from build123d import *

# Parameters (mm, degrees)
SKETCH_W        = 76.2
SKETCH_H        = 76.2
PAD_DEPTH       = 4
SKETCH001_R     = 25.4
POCKET_DEPTH    = 4.001
SKETCH002_R     = 2.25
POCKET001_DEPTH = 4.001
SKETCH003_R     = 30.4
SKETCH003_R_2   = 25.4
PAD001_DEPTH    = 25
SKETCH004_R     = 30.4
PAD002_DEPTH    = 3
SKETCH005_W     = 6
SKETCH005_H     = 11
POCKET002_DEPTH = 32.001
SKETCH006_W     = 5
SKETCH006_H     = 38
PAD003_DEPTH    = 42
POCKET003_DEPTH = 33.351
FILLET_R        = 1.5
FILLET001_R     = 3
FILLET002_R     = 0.4
FILLET003_R     = 3
FILLET004_R     = 6


with BuildPart() as part:
    # Sketch → Pad (new body)
    with BuildSketch(Plane.XY):
        Rectangle(SKETCH_W, SKETCH_H)
    extrude(amount=PAD_DEPTH)

    # Sketch001 (on Face6 of Pad) → Pocket (cut, through all)
    with BuildSketch(Plane.XY.offset(4)):
        Circle(SKETCH001_R)
    extrude(amount=-POCKET_DEPTH, mode=Mode.SUBTRACT)

    # Sketch002 (on Face5 of Pocket) → Pocket001 (cut, through all)
    with BuildSketch(Plane.XY.offset(4)):
        with Locations((-30.1, -30.1)):
            Circle(SKETCH002_R)
        with Locations((30.1, -30.1)):
            Circle(SKETCH002_R)
        with Locations((30.1, 30.1)):
            Circle(SKETCH002_R)
        with Locations((-30.1, 30.1)):
            Circle(SKETCH002_R)
    extrude(amount=-POCKET001_DEPTH, mode=Mode.SUBTRACT)

    # Sketch003 (on Face5 of Pocket001) → Pad001 (join)
    with BuildSketch(Plane.XY.offset(4)):
        Circle(SKETCH003_R)
        Circle(SKETCH003_R_2, mode=Mode.SUBTRACT)
    extrude(amount=PAD001_DEPTH)

    # Sketch004 (on Face14 of Pad001) → Pad002 (join)
    with BuildSketch(Plane.XY.offset(29)):
        Circle(SKETCH004_R)
    extrude(amount=PAD002_DEPTH)

    # Sketch005 (on Face16 of Pad002) → Pocket002 (cut, through all)
    with BuildSketch(Plane.XY.offset(32)):
        Rectangle(SKETCH005_W, SKETCH005_H)
    extrude(amount=-POCKET002_DEPTH, mode=Mode.SUBTRACT)

    # Sketch006 (on Face16 of Pocket002) → Pad003 (join)
    with BuildSketch(Plane.XY.offset(32)):
        with Locations((7.25, -8)):
            Rectangle(SKETCH006_W, SKETCH006_H)
    extrude(amount=PAD003_DEPTH)

    # CopySketch007 (on Face21 of Pad003) → Pocket003 (cut, through all)
    with BuildSketch(Plane(origin=(4.75, 0, 0), x_dir=(0, -1, 0), z_dir=(-1, 0, 0))):
        with BuildLine():
            ThreePointArc((-5.25, 45.013309), (-3, 42.763309), (-0.75, 45.013309))
            Line((-0.75, 45.013309), (-0.75, 70.013309))
            ThreePointArc((-0.75, 70.013309), (-3, 72.263309), (-5.25, 70.013309))
            Line((-5.25, 45.013309), (-5.25, 70.013309))
        make_face()
        with BuildLine():
            ThreePointArc((17.25, 35.513309), (19.5, 33.263309), (21.75, 35.513309))
            Line((21.75, 35.513309), (21.75, 60.513309))
            ThreePointArc((21.75, 60.513309), (19.5, 62.763309), (17.25, 60.513309))
            Line((17.25, 35.513309), (17.25, 60.513309))
        make_face()
    extrude(amount=-POCKET003_DEPTH, mode=Mode.SUBTRACT)

    # Fillet
    fillet_edges = [part.edges().sort_by_distance(p)[0] for p in [
        (4.75, -8, 32),
    ]]
    fillet(fillet_edges, radius=FILLET_R)

    # Fillet001
    fillet001_edges = [part.edges().sort_by_distance(p)[0] for p in [
        (9.75, -8, 32),
    ]]
    fillet(fillet001_edges, radius=FILLET001_R)

    # Fillet002
    fillet002_edges = [part.edges().sort_by_distance(p)[0] for p in [
        (7.25, -27, 32),
    ]]
    fillet(fillet002_edges, radius=FILLET002_R)

    # Fillet003
    fillet003_edges = [part.edges().sort_by_distance(p)[0] for p in [
        (7.25, 11, 32),
    ]]
    fillet(fillet003_edges, radius=FILLET003_R)

    # Fillet004
    fillet004_edges = [part.edges().sort_by_distance(p)[0] for p in [
        (7.25, -27, 74),
        (7.25, 11, 74),
    ]]
    fillet(fillet004_edges, radius=FILLET004_R)


solid = part.part
Verification items for the finished model (mm, model axes). A direction names the side the tool comes from. Coordinates: 2 decimals unless noted, no trailing zeros. Write each loop counter-clockwise with the first axis right and the second up, starting at its lowest first coordinate (ties: lowest second). Pieces come first, ordered by that corner, then holes. Notation, with made-up numbers: M -27,43 L 8,43 A15 ccw 8,53 Z; hole C 25,75.5 d3. An arc over 180 degrees is marked long. Use a Markdown table: item, result.
Q1. Thickness scan on line 1 (X direction, y = -30, z = 1); line 2 (Y direction, x = 8, z = 47). Record the ranges inside material, lowest first.
Reply:
| item | result |
|---|---|
| line 1 | x = -38.1 to -32.35, -27.85 to 27.85, 32.35 to 38.1 |
| line 2 | y = -27 to -21.75, -17.25 to 0.75, 5.25 to 11 |
Q2. Sectioned sample at C-C, the plane y = 3. Record the boundary of the cut face in (x, z), plus the area to 3 significant figures.
Reply:
| item | result |
|---|---|
| outline | M -38.1,0 L -25.22,0 L -25.22,29 L -3,29 L -3,32 L -30.25,32 L -30.25,4 L -38.1,4 Z; M 3,29 L 25.22,29 L 25.22,0 L 38.1,0 L 38.1,4 L 30.25,4 L 30.25,32 L 12.75,32 A3 cw 9.75,35 L 9.75,42.76 L 4.75,42.76 L 4.75,33.5 A1.5 cw 3.25,32 L 3,32 Z; M 4.75,72.26 L 9.75,72.26 L 9.75,74 L 4.75,74 Z |
| area | 583 mm² |
Q3. Draft check along X on faces 1 (the face through (7.285, 9.196, 72.289)), 2 (the face through (29.81, -27.87, 2.03)), 3 (the face through (-30.37, 1.34, 17.8)). Enter one of: +X half, -X half, draft (parallel to the pull), parting line (faces both ways), or undercut.
Reply:
| item | result |
|---|---|
| face 1 | draft |
| face 2 | undercut |
| face 3 | parting line |
Q4. Sectioned sample at A-A, the plane x = 0. Record the boundary of the cut face in (y, z).
Reply:
| item | result |
|---|---|
| outline | M -38.1,0 L -25.4,0 L -25.4,29 L -5.5,29 L -5.5,32 L -30.4,32 L -30.4,4 L -38.1,4 Z; M 5.5,29 L 25.4,29 L 25.4,0 L 38.1,0 L 38.1,4 L 30.4,4 L 30.4,32 L 5.5,32 Z |
Q5. Sectioned sample at B-B, the plane z = 41.5. Record the boundary of the cut face in (x, y), plus the area to 4 significant figures.
Reply:
| item | result |
|---|---|
| outline | M 4.75,-27 L 9.75,-27 L 9.75,-21.75 L 4.75,-21.75 Z; M 4.75,-17.25 L 9.75,-17.25 L 9.75,11 L 4.75,11 Z |
| area | 167.5 mm² |
Q6. Go/stop test with flat-tipped pins: P1, Ø5, axis at x = 5, z = 59, coming from the -Y side; P2, Ø0.9, axis at y = 0, z = 31, coming from the +X side; P3, Ø1, axis at x = -21.5, z = 8.5, coming from the +Y side; P4, Ø3, axis at x = -25.5, y = -21, coming from the -Z side. Record where each tip stops, or that it passes through.
Reply:
| item | result |
|---|---|
| P1 | stops at y = -27 |
| P2 | stops at x = 30.4 |
| P3 | stops at y = 21.98 |
| P4 | stops at z = 0 |
Q7. Sectioned sample at D-D, the plane z = 9. Record the boundary of the cut face in (x, y).
Reply:
| item | result |
|---|---|
| outline | C 0,0 d60.8; hole C 0,0 d50.8 |
Q8. Set-up check for faces 4 (the face through (-26, 17, 4)), 5 (the face through (7, 0.75, 57)), 6 (the face through (5, 0, 29)), 7 (the face through (3, 0, 31)): record each of +Z, -Z, +X, -X, +Y, -Y from which the full face is reachable in a straight line by a thin tool's end or side.
Reply:
| item | result |
|---|---|
| face 4 | +Z |
| face 5 | +X, -X |
| face 6 | -Z |
| face 7 | +Z, -Z |
